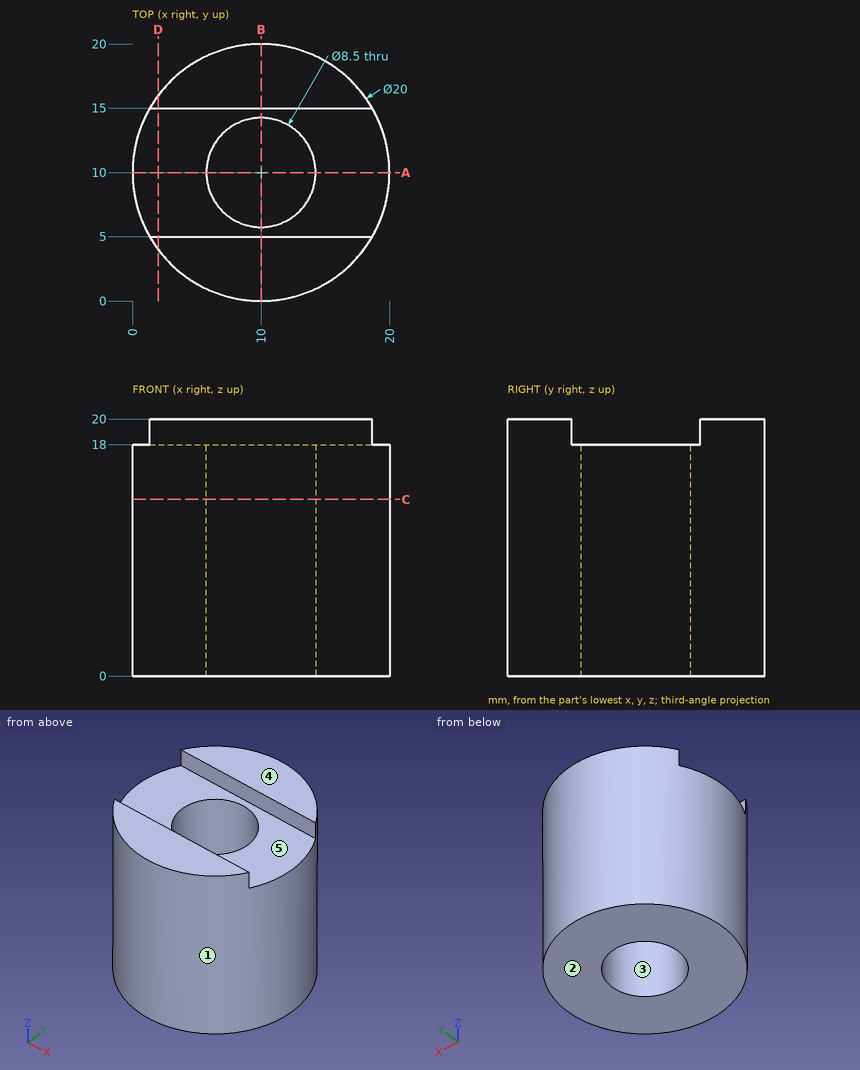
Design review of the part shown in the three views and the two pictorial views. Dimensions are in mm from the part's minimum x, y and z. A direction names the side the tool comes from. Round coordinates to 2 decimals unless told otherwise and drop trailing zeros. Order: outer loops, then holes, each group sorted by start corner. A loop starts at its lowest first (then second) coordinate and runs counter-clockwise, first axis right, second up. Notation, with made-up numbers: (58.25, 39.25) - (77.25, 39.25) arc R14 ccw to (77.25, 62.25) - close; hole circle Ø1 at (34, 12.5). An arc over 180 degrees is marked (long way). One line per question, with ' | ' between items.
Item 1: Take a section at A-A, the plane y = 10. Write out the cut boundary in (x, z).
Checks:
outline: (0, 0) - (5.75, 0) - (5.75, 18) - (0, 18) - close; (14.25, 0) - (20, 0) - (20, 18) - (14.25, 18) - close
Item 2: Take a section at C-C, the plane z = 13.75. Write out the cut boundary in (x, y), then the cut area to 3 significant figures.
Checks:
outline: circle Ø20 at (10, 10); hole circle Ø8.5 at (10, 10) | area: 257 mm²
Item 3: Take a section at B-B, the plane x = 10. Write out the cut boundary in (y, z).
Checks:
outline: (0, 0) - (5.75, 0) - (5.75, 18) - (5, 18) - (5, 20) - (0, 20) - close; (14.25, 0) - (20, 0) - (20, 20) - (15, 20) - (15, 18) - (14.25, 18) - close
Item 4: Wall thickness on line 1 (Y direction, x = 10, z = 11.75); line 2 (Z direction, x = 19, y = 10.5); line 3 (X direction, y = 5, z = 12.5): over which ranges is each line inside the solid? List them lowest first. Write a range as [from, to].
Checks:
line 1: [0, 5.75], [14.25, 20] | line 2: [0, 18] | line 3: [1.34, 18.66]
Item 5: Draft analysis for pull direction X (two halves, no side actions). For the marked faces 1, 2 and 3, state which applies: +X half, -X half, draft (parallel to the pull), parting line (faces both ways), or undercut.
Checks:
face 1: parting line | face 2: draft | face 3: undercut
Item 6: Take a section at D-D, the plane x = 2. Write out the cut boundary in (y, z), then the cut area to 3 significant figures.
Checks:
outline: (4, 0) - (16, 0) - (16, 20) - (15, 20) - (15, 18) - (5, 18) - (5, 20) - (4, 20) - close | area: 220 mm²
Item 7: For P1, Ø2, axis at x = 7.5, z = 19, coming from the +Y side; P2, Ø10, axis at y = 4.5, z = 12, coming from the +X side; P3, Ø3, axis at x = 13, y = 9.5, coming from the +Z side, all flat-tipped, find the tip position at first contact; note any pin that passes through.
Checks:
P1: y = 19.89 | P2: x = 19.99 | P3: z = 18
Item 8: Machinability: for the marked faces 4 and 5, which of the approach directions +Z, -Z, +X, -X, +Y, -Y give a long, thin tool a straight path to every point of the face, cutting with its end or side? Answer none if there is none.
Checks:
face 4: +Z, +X, -X, +Y, -Y | face 5: +Z, +X, -X
